```python
from build123d import *

# Parameters (mm, degrees)
EXTRUDE_5_DEPTH     = 20
SKETCH_4_R          = 1.55
CUT_EXTRUDE_1_DEPTH = 10
CUT_EXTRUDE_2_DEPTH = 5
CUT_EXTRUDE_START   = -5
CUT_EXTRUDE_3_DEPTH = 5
CUT_EXTRUDE_4_DEPTH = 5
EXTRUDE_7_DEPTH     = 20
CUT_EXTRUDE_6_DEPTH = 30
CUT_EXTRUDE_START_2 = -10
SKETCH_11_R         = 1
CUT_EXTRUDE_7_DEPTH = 10
EXTRUDE_8_DEPTH     = 10


with BuildPart() as part:
    # Sketch 1 → Extrude 5 (new body)
    with BuildSketch(Plane(origin=(0, 0, 0), x_dir=(1, 0, 0), z_dir=(0, 1, 0))):
        with BuildLine():
            Line((-9.02810898, 9.014963713), (-9.601685416, 8.195811669))
            Line((-9.601685416, 8.195811669), (-7.553805305, 6.761870578))
            ThreePointArc((-7.553805305, 6.761870578), (4.479399484, -61.481824974), (-63.764296068, -73.515029763))
            Line((-63.764296068, -73.515029763), (-66.058601813, -76.79163794))
            ThreePointArc((-66.058601813, -76.79163794), (6.240788915, -65.832756837), (-1.221646395, 6.910703583))
            Line((-1.221646395, 6.910703583), (18.546430176, 33.576189082))
            Line((18.546430176, 33.576189082), (19.730587978, 35.267341687))
            ThreePointArc((19.730587978, 35.267341687), (19.896243687, 36.014566301), (19.48501237, 36.660070167))
            Line((19.48501237, 36.660070167), (13.341372038, 40.96189344))
            Line((13.341372038, 40.96189344), (-7.880956107, 10.653267801))
            Line((-7.880956107, 10.653267801), (-8.454532543, 9.834115757))
            Line((-8.454532543, 9.834115757), (-9.02810898, 9.014963713))
        make_face()
    extrude(amount=EXTRUDE_5_DEPTH)

    # Sketch 4 → Cut-Extrude 1 (cut)
    with BuildSketch(Plane(origin=(-10.293599492, 0, -7.20765596), x_dir=(-0.5735764363510502, 0, 0.8191520442889891), z_dir=(-0.8191520442889891, 0, -0.5735764363510502))):
        with Locations((-36.406315379, 14.8)):
            Circle(SKETCH_4_R)
        with Locations((-36.406315379, 5.2)):
            Circle(SKETCH_4_R)
    extrude(amount=-CUT_EXTRUDE_1_DEPTH, mode=Mode.SUBTRACT)

    # Sketch 4_4 → Cut-Extrude 2 (cut)
    with BuildSketch(Plane(origin=(-10.293599492, 0, -7.20765596), x_dir=(-0.5735764363510502, 0, 0.8191520442889891), z_dir=(-0.8191520442889891, 0, -0.5735764363510502))):
        Polygon((-34.71546965, 11.84291122), (-32.99997851, 14.785770965), (-34.690824239, 17.742859745), (-38.097161108, 17.75708878), (-39.812652248, 14.814229035), (-38.121806519, 11.857140255), align=None)
        Polygon((-34.611807013, 2.304646298), (-33.001611337, 5.306412981), (-34.796119703, 8.201766683), (-38.200823744, 8.095353702), (-39.811019421, 5.093587019), (-38.016511055, 2.198233317), align=None)
    extrude(amount=-CUT_EXTRUDE_2_DEPTH, mode=Mode.SUBTRACT)

    # Sketch 5 → Cut-Extrude 3 (cut)
    with BuildSketch(Plane(origin=(0, 20, 0), x_dir=(1, 0, 0), z_dir=(0, 1, 0)).offset(CUT_EXTRUDE_START)):
        with BuildLine():
            Line((-7.553805305, 6.761870578), (-1.221646395, 6.910703583))
            ThreePointArc((-1.221646395, 6.910703583), (6.240788915, -65.832756837), (-66.058601813, -76.79163794))
            Line((-66.058601813, -76.79163794), (-63.764296068, -73.515029763))
            ThreePointArc((-63.764296068, -73.515029763), (4.479399484, -61.481824974), (-7.553805305, 6.761870578))
        make_face()
    extrude(amount=CUT_EXTRUDE_3_DEPTH, mode=Mode.SUBTRACT)

    # Sketch 6 → Cut-Extrude 4 (cut)
    with BuildSketch(Plane.XZ):
        with BuildLine():
            Line((-7.553805305, -6.761870578), (-1.221646395, -6.910703583))
            ThreePointArc((-1.221646395, -6.910703583), (6.240788915, 65.832756837), (-66.058601813, 76.79163794))
            Line((-66.058601813, 76.79163794), (-63.764296068, 73.515029763))
            ThreePointArc((-63.764296068, 73.515029763), (4.479399484, 61.481824974), (-7.553805305, -6.761870578))
        make_face()
    extrude(amount=-CUT_EXTRUDE_4_DEPTH, mode=Mode.SUBTRACT)

    # Sketch 9 → Extrude 7 (add)
    with BuildSketch(Plane(origin=(0, 0, 0), x_dir=(1, 0, 0), z_dir=(0, 1, 0))):
        Polygon((8.662391891, 20.243446333), (-1.221646395, 6.910703583), (8.662391891, -5.275766787), align=None)
    extrude(amount=EXTRUDE_7_DEPTH)

    # Sketch 7 → Cut-Extrude 6 (cut)
    with BuildSketch(Plane(origin=(-10.293599492, 0, -7.20765596), x_dir=(-0.5735764363510472, 0, 0.819152044288991), z_dir=(-0.819152044288991, 0, -0.5735764363510472))):
        Polygon((-1.206315379, 5), (-16.473642116, 0), (0, 0), (28.572588785, 0), (28.572588785, 5), align=None)
        Polygon((-1.206315379, 20), (-16.473642116, 20), (-1.206315379, 15), (28.572588785, 15), (28.572588785, 20), align=None)
    extrude(amount=-CUT_EXTRUDE_6_DEPTH, mode=Mode.SUBTRACT)

    # Sketch 11 → Cut-Extrude 7 (cut)
    with BuildSketch(Plane(origin=(0, 15, 0), x_dir=(1, 0, 0), z_dir=(0, 1, 0)).offset(CUT_EXTRUDE_START_2)):
        with Locations((-34.481669179, -37.284707791)):
            Circle(SKETCH_11_R)
        with BuildLine():
            Line((-63.764296068, -73.515029763), (-66.058601813, -76.79163794))
            ThreePointArc((-66.058601813, -76.79163794), (-53.786118283, -83.180288494), (-40.278305052, -86.174898591))
            Line((-40.278305052, -86.174898591), (-39.929682081, -82.190119799))
            ThreePointArc((-39.929682081, -82.190119799), (-52.41803771, -79.421518011), (-63.764296068, -73.515029763))
        make_face()
    extrude(amount=CUT_EXTRUDE_7_DEPTH, mode=Mode.SUBTRACT)

    # Sketch 18 → Extrude 8 (add)
    with BuildSketch(Plane(origin=(0, 15, 0), x_dir=(1, 0, 0), z_dir=(0, 1, 0))):
        with BuildLine():
            ThreePointArc((-39.929682081, -82.190119799), (-42.096382963, -84.00819771), (-40.278305052, -86.174898591))
            Line((-40.278305052, -86.174898591), (-39.929682081, -82.190119799))
        make_face()
    extrude(amount=-EXTRUDE_8_DEPTH)


solid = part.part
```
Work out the finished part from the listing and answer in its coordinate system (mm). A direction names the side the tool comes from. Coordinates: 2 decimals unless noted, no trailing zeros. Write each loop counter-clockwise with the first axis right and the second up, starting at its lowest first coordinate (ties: lowest second). Pieces come first, ordered by that corner, then holes.
Q1. Each of these flat-tipped pins is pushed along its axis until it touches: pin 1 Ø6 at (y, z) = (4.5, -26) entering from -X; pin 2 Ø6 at (y, z) = (17, 0) entering from +X; pin 3 Ø4 at (y, z) = (11, -21.5) entering from -X; pin 4 Ø2 at (y, z) = (2.5, 6) entering from -X. Where does it stop, or does it pass through?
Q2. A cutting plane is placed at B-B, the plane y = 10.5. Give the vertices of the cut face in (x, z), then the cut area to 3 significant figures.
Q3. Which of the six approach directions +Z, -Z, +X, -X, +Y, -Y give full straight-line access (tool end or side, diameter ignored) to faces 1 (the face through (14.092, 6.615, -37.736)), 2 (the face through (13.54, 9.86, -26.82)), 3 (the face through (11.1, 3.8, -33.5))?
Q4. Determine the mould class of faces 4 (the face through (2.063, 15.469, -2.86)), 5 (the face through (16.46, 9.86, -38.78)), 6 (the face through (15.58, 15.5, -35.44)) for opening direction Z: released by +Z, released by -Z, zero draft, split by the parting line, or undercut.
Q5. A cutting plane is placed at C-C, the plane z = 22.5. Give the vertices of the cut face in (x, y), then the cut area to 3 significant figures.
Q6. A cutting plane is placed at D-D, the plane x = -17.5. Give the vertices of the cut face in (y, z), then the cut area to 3 significant figures.
Q7. Find the intervals of material crossed by line 1 (Z direction, x = 13, y = 17.5); line 2 (Z direction, x = 3, y = 13); line 3 (Z direction, x = 10.5, y = 17), in increasing order.
Q8. A cutting plane is placed at A-A, the plane x = 2. Give the vertices of the cut face in (y, z), then the cut area to 3 significant figures.
Findings below:
1. pin 1: stops at x = 0.76
1. pin 2: stops at x = 8.66
1. pin 3: stops at x = -1.69
1. pin 4: passes through
2. outline: (-40.28, 86.17) arc R2 ccw to (-39.93, 82.19) arc R49 cw to (-7.55, -6.76) - (-9.6, -8.2) - (13.34, -40.96) - (19.49, -36.66) arc R1 ccw to (19.73, -35.27) - (18.55, -33.58) - (8.66, -20.24) - (8.66, 4.31) arc R53 ccw to start
2. area: 958 mm2
3. face 1: -X
3. face 2: +X, +Y, -Y
3. face 3: none
4. face 4: released by +Z
4. face 5: released by -Z
4. face 6: undercut
5. outline: (12.12, 5) - (16.21, 5) - (16.21, 15) - (12.12, 15) - close
5. area: 40.9 mm2
6. outline: (5, 78.89) - (15, 78.89) - (15, 83.17) - (5, 83.17) - close
6. area: 42.8 mm2
7. line 1: z = -40.47 to -37.59, -33.08 to -26.09
7. line 2: z = -26.19 to 3.27, 63.48 to 69.63
7. line 3: z = -34.48 to -22.72
8. outline: (0, -24.76) - (20, -24.76) - (20, -18.71) - (15.77, -2.94) - (15, -2.94) - (15, 2.03) - (5, 2.03) - (5, -2.94) - (4.23, -2.94) - (0, -18.71) - close; (5, 64.73) - (15, 64.73) - (15, 70.67) - (5, 70.67) - close
8. area: 479 mm2
